Work out the finished part from the listing and answer in its coordinate system (mm). A direction names the side the tool comes from. Coordinates: 2 decimals unless noted, no trailing zeros. Order: outer loops, then holes, each group sorted by start corner. A loop starts at its lowest first (then second) coordinate and runs counter-clockwise, first axis right, second up. Notation, with made-up numbers: (49.5, 35) -> (63.5, 35) arc R16 ccw to (63.5, 43) -> close; hole circle Ø1 at (-28, -11.5). An arc over 180 degrees is marked (long way). Write item = value, one per line. Start each with the question number.
Q1. Flat-ended cylindrical pins translate along their axes: pin 1 (15 mm diameter, centred on x = -43.5, y = -5.5, fed in from +Z); pin 2 (0.6 mm diameter, centred on y = -30.5, z = 18.5, fed in from -X); pin 3 (5 mm diameter, centred on x = -33, z = 20.5, fed in from +Y) (3 decimals); pin 4 (1.5 mm diameter, centred on x = -23.5, z = 20, fed in from +Y). Find the tip coordinate at first contact, or state that the pin passes through.
Q2. Which of the six approach directions +Z, -Z, +X, -X, +Y, -Y give full straight-line access (tool end or side, diameter ignored) to faces 4 (the flat face through (-67, -31, 23.622)), 5 (the flat face through (-38.43, -12.08, 13.4)), 6 (the cylindrical face through (-4.066, -3.899, 18.166))?
Q3. For a pull along Y with two mould halves and no side action, classify faces 1 (the cylindrical face through (-3.264, -34.161, 18.166)), 2 (the flat face through (-41, -36, 17.78)), 3 (the cylindrical face through (-7.653, -8.067, 20.671)) as +Y half, -Y half, draft (parallel to the pull), parting line (faces both ways), or undercut.
Q4. The part is cut by section B-B, the plane x = -29.5. Determine the outline of the cut face in (y, z) (3 decimals), plus the area to 3 significant figures.
Q5. The part is cut by section A-A, the plane z = 20. Determine the outline of the cut face in (x, y) (3 decimals), plus the area to 3 significant figures.
Q6. Straight lines are drawn through the part: L1, parallel to Z at x = -66.5, y = -12.5; L2, parallel to Z at x = -4.5, y = -34; L3, parallel to Y at x = -59.5, z = 9.75 (3 decimals). For each, find the intervals that lie inside material, in ascending order. Write a range as from..to.
Q7. The part is cut by section D-D, the plane x = -57.5. Determine the outline of the cut face in (y, z) (3 decimals).
Q8. The part is cut by section C-C, the plane y = -20. Determine the outline of the cut face in (x, z), plus the area to 3 significant figures.
```python
from build123d import *

# Parameters (mm, degrees)
SKETCH1_W           = 76.2
SKETCH1_H           = 38.1
BOSS_EXTRUDE1_DEPTH = 17.78
CUT_EXTRUDE1_DEPTH  = 8.89
FILLET1_R           = 3.175
SKETCH3_R           = 2.54
BOSS_EXTRUDE2_DEPTH = 5.842
CHAMFER1_SIZE       = 0.762
BOSS_EXTRUDE3_DEPTH = 0.762
FILLET2_R           = 2.54
BOSS_EXTRUDE4_DEPTH = 0.762
FILLET3_R           = 2.54


with BuildPart() as part:
    # Sketch1 → Boss-Extrude1 (new body)
    with BuildSketch(Plane.XY):
        with Locations((-38.1, -19.05)):
            Rectangle(SKETCH1_W, SKETCH1_H)
    extrude(amount=BOSS_EXTRUDE1_DEPTH)

    # Sketch2 → Cut-Extrude1 (cut)
    with BuildSketch(Plane.XY.offset(17.78)):
        Polygon((-76.2, -24.13), (-76.2, -13.97), (0, -10.16), (0, -27.94), align=None)
    extrude(amount=-CUT_EXTRUDE1_DEPTH, mode=Mode.SUBTRACT)

    # Fillet1
    fillet1_edges = [part.edges().sort_by_distance(p)[0] for p in [
        (-76.2, -13.97, 13.335),
        (0, -10.16, 13.335),
        (0, -27.94, 13.335),
        (-76.2, -24.13, 13.335),
    ]]
    fillet(fillet1_edges, radius=FILLET1_R)

    # Sketch3 → Boss-Extrude2 (add)
    with BuildSketch(Plane.XY.offset(17.78)):
        with Locations(Location((-9.525, -6.35, 0), (0, 0, 180))):
            Circle(SKETCH3_R)
        with Locations(Location((-66.675, -31.369, 0), (0, 0, 180))):
            Circle(SKETCH3_R)
    extrude(amount=BOSS_EXTRUDE2_DEPTH)

    # Chamfer1
    chamfer1_edges = [part.edges().sort_by_distance(p)[0] for p in [
        (-6.985, -6.35, 23.622),
        (-64.135, -31.369, 23.622),
    ]]
    chamfer(chamfer1_edges, length=CHAMFER1_SIZE)

    # Sketch4 → Boss-Extrude3 (add)
    with BuildSketch(Plane.XY.offset(17.78)):
        Polygon((-73.66, -26.035), (-2.54, -29.083), (-2.54, -34.925), (-73.66, -34.925), align=None)
    extrude(amount=BOSS_EXTRUDE3_DEPTH)

    # Fillet2
    fillet2_edges = [part.edges().sort_by_distance(p)[0] for p in [
        (-73.66, -26.035, 18.161),
        (-73.66, -34.925, 18.161),
        (-2.54, -34.925, 18.161),
        (-2.54, -29.083, 18.161),
    ]]
    fillet(fillet2_edges, radius=FILLET2_R)

    # Sketch5 → Boss-Extrude4 (add)
    with BuildSketch(Plane.XY.offset(17.78)):
        Polygon((-73.192591087, -3.175), (-3.302, -3.175), (-3.302, -9.525), (-73.192591087, -12.065), align=None)
    extrude(amount=BOSS_EXTRUDE4_DEPTH)

    # Fillet3
    fillet3_edges = [part.edges().sort_by_distance(p)[0] for p in [
        (-73.192591087, -3.175, 18.161),
        (-73.192591087, -12.065, 18.161),
        (-3.302, -9.525, 18.161),
        (-3.302, -3.175, 18.161),
    ]]
    fillet(fillet3_edges, radius=FILLET3_R)


solid = part.part
```
Model answer:
q1.pin_1 = 18.54
q1.pin_2 = -73.66
q1.pin_3 = -3.175
q1.pin_4 = through
q2.face_4 = +Z, +X, -X, +Y, -Y
q2.face_5 = +Z, +X
q2.face_6 = +Z, +X, +Y
q3.face_1 = -Y half
q3.face_2 = undercut
q3.face_3 = parting line
q4.outline = (-38.1, 0) -> (0, 0) -> (0, 17.78) -> (-3.175, 17.78) -> (-3.175, 18.542) -> (-10.477, 18.542) -> (-10.477, 17.78) -> (-11.635, 17.78) -> (-11.635, 8.89) -> (-26.465, 8.89) -> (-26.465, 17.78) -> (-27.928, 17.78) -> (-27.928, 18.542) -> (-34.925, 18.542) -> (-34.925, 17.78) -> (-38.1, 17.78) -> close
q4.area = 556 mm2
q5.outline = circle Ø5.08 at (-66.675, -31.369); circle Ø5.08 at (-9.525, -6.35)
q5.area = 40.5 mm2
q6.L1 = 0..17.78
q6.L2 = 0..18.54
q6.L3 = -38.1..-24.965, -13.135..0
q7.outline = (-38.1, 0) -> (0, 0) -> (0, 17.78) -> (-3.175, 17.78) -> (-3.175, 18.542) -> (-11.495, 18.542) -> (-11.495, 17.78) -> (-13.035, 17.78) -> (-13.035, 8.89) -> (-25.065, 8.89) -> (-25.065, 17.78) -> (-26.728, 17.78) -> (-26.728, 18.542) -> (-34.925, 18.542) -> (-34.925, 17.78) -> (-38.1, 17.78) -> close
q8.outline = (-76.2, 0) -> (0, 0) -> (0, 8.89) -> (-76.2, 8.89) -> close
q8.area = 677 mm2
